from build123d import *

# Parameters (mm, degrees)
F0_R      = 35.543794
F1_DEPTH  = 100
F2_R      = 16.15749
F3_DEPTH  = 25.4
F1_FACE_R = 35.543794
F4_DEPTH  = 25.4


with BuildPart() as f1:
    # F0 (on Top) → F1 (new body)
    with BuildSketch(Plane.XY):
        with Locations((0, 0.879988)):
            Circle(F0_R)
    extrude(amount=F1_DEPTH)

    # F2 (on face) → F3 (join)
    with BuildSketch(Plane.XY.offset(100)):
        Circle(F2_R)
    extrude(amount=-F3_DEPTH)

    # F1_face (on face) → F4 (join)
    with BuildSketch(Plane(origin=(0, 0.879988, 100), x_dir=(1, 0, 0), z_dir=(0, 0, 1))):
        Circle(F1_FACE_R)
    extrude(amount=F4_DEPTH)


solid = f1.part
Read the model definition and answer for the solid it produces. Units are mm, in the model's axes. Give positions to 0.01 mm unless a question says otherwise; leave off trailing zeros. Write each loop counter-clockwise with the first axis right and the second up, starting at its lowest first coordinate (ties: lowest second). Pieces come first, ordered by that corner, then holes. Notation, with made-up numbers: (81, 64.5) - (140, 64.5) arc R8 ccw to (140, 77.5) - close; hole circle Ø5 at (-1.75, -21.75). An arc over 180 degrees is marked (long way). Use CSV: the item, a comma, the result in double quotes. Start each with the question number.
Item 1: The part is cut by section B-B, the plane y = 9. Give the vertices of the cut face in (x, z).
Item 2: The part is cut by section C-C, the plane z = 111. Give the vertices of the cut face in (x, y), and give its area (3 significant figures).
Item 3: Consider line 1 (X direction, y = 1.5, z = 28); line 2 (Y direction, x = 32, z = 74); line 3 (Y direction, x = -1, z = 83). Determine where each line is inside the solid, lowest interval first.
Item 4: Flat-ended cylindrical pins translate along their axes: P1, Ø1.5, axis at x = -28.5, z = 32, coming from the -Y side; P2, Ø10, axis at x = 6.5, z = 83, coming from the +Y side; P3, Ø8, axis at y = 29, z = 93, coming from the -X side. Find the tip coordinate at first contact, or state that the pin passes through.
Item 5: The part is cut by section A-A, the plane x = -29.5. Give the vertices of the cut face in (y, z).
Taken from the geometry:
1,outline,"(-34.6, 0) - (34.6, 0) - (34.6, 125.4) - (-34.6, 125.4) - close"
2,outline,"circle Ø71.09 at (0, 0.88)"
2,area,"3,970 mm2"
3,line 1,"-35.54 to 35.54"
3,line 2,"-14.59 to 16.35"
3,line 3,"-34.65 to 36.41"
4,P1,"y = -21.33"
4,P2,"y = 36.39"
4,P3,"x = -26.11"
5,outline,"(-18.95, 0) - (20.71, 0) - (20.71, 125.4) - (-18.95, 125.4) - close"
